Geometry: final body of the model. Coordinates: model frame, mm. A direction names the side the tool comes from. Coordinates: 2 decimals unless noted, no trailing zeros. Write each loop counter-clockwise with the first axis right and the second up, starting at its lowest first coordinate (ties: lowest second). Pieces come first, ordered by that corner, then holes. Notation, with made-up numbers: (53.5, 40.25) - (62.5, 40.25) arc R14 ccw to (62.5, 56.25) - close; hole circle Ø9 at (1.5, 83.5). An arc over 180 degrees is marked (long way). Put each result on its own line as item: value.
```python
from build123d import *

# Parameters (mm, degrees)
SKETCH1_W              = 250
SKETCH1_H              = 358.226
BASE_FLANGE1_DEPTH     = 0.91
SKETCHED_START         = -125
SKETCHED_BEND1_DEPTH   = 250
SKETCHED_BEND1_2_DEPTH = 250
SKETCH10_R             = 2.35
CUT_EXTRUDE1_DEPTH     = 0.91
FILLET1_R              = 1.5
SKETCH11_R             = 2.35
CUT_EXTRUDE2_DEPTH     = 10
SKETCH12_R             = 1.7
SKETCH12_W             = 30.3
SKETCH12_H             = 22.3
CUT_EXTRUDE3_DEPTH     = 10
FILLET2_R              = 5


# Read off the part's stored shape, not the designer's step: Sketched Bend1
# Sheet-metal steps are written as plain solids
with BuildPart() as part:
    # Sketch1 → Base-Flange1 (new body)
    with BuildSketch(Plane(origin=(0, 0, 0), x_dir=(1, 0, 0), z_dir=(0, 1, 0))):
        Rectangle(SKETCH1_W, SKETCH1_H)
    extrude(amount=-BASE_FLANGE1_DEPTH)

    # Sketched Bend1 outline → Sketched Bend1 (cut)
    with BuildSketch(Plane.YZ.offset(SKETCHED_START)):
        with BuildLine():
            ThreePointArc((-0.91, 68.830699214), (-0.668268616, 69.797195464), (0, 70.536090665))
            Line((0, 70.536090665), (0, 179.113))
            Line((0, 179.113), (-0.91, 179.113))
            Line((-0.91, 179.113), (-0.91, 68.830699214))
        make_face()
    extrude(amount=SKETCHED_BEND1_DEPTH, mode=Mode.SUBTRACT)

    # Sketched Bend1 2 outline → Sketched Bend1 2 (add)
    with BuildSketch(Plane.YZ.offset(SKETCHED_START)):
        with BuildLine():
            Line((109.086699214, 69.973699214), (109.086699214, 70.883699214))
            Line((109.086699214, 70.883699214), (1.143, 70.883699214))
            ThreePointArc((1.143, 70.883699214), (0.545655731, 70.794875587), (0, 70.536090665))
            Line((0, 70.536090665), (0, 68.830699214))
            ThreePointArc((0, 68.830699214), (0.334776949, 69.638922265), (1.143, 69.973699214))
            Line((1.143, 69.973699214), (109.086699214, 69.973699214))
        make_face()
    extrude(amount=SKETCHED_BEND1_2_DEPTH)

    # Sketch10 → Cut-Extrude1 (cut)
    with BuildSketch(Plane(origin=(0, 0, 0), x_dir=(1, 0, 0), z_dir=(0, 1, 0))):
        with Locations(Location((-105, 159.113, 0), (0, 0, 270))):
            Circle(SKETCH10_R)
        with Locations(Location((105, 159.113, 0), (0, 0, 270))):
            Circle(SKETCH10_R)
        with Locations(Location((105, -50.883699214, 0), (0, 0, 270))):
            Circle(SKETCH10_R)
        with Locations(Location((-105, -50.883699214, 0), (0, 0, 270))):
            Circle(SKETCH10_R)
    extrude(amount=-CUT_EXTRUDE1_DEPTH, mode=Mode.SUBTRACT)

    # Fillet1
    fillet1_edges = [part.edges().sort_by_distance(p)[0] for p in [
        (-125, -0.455, -179.113),
        (125, -0.455, -179.113),
        (125, 109.086699214, 70.428699214),
        (-125, 109.086699214, 70.428699214),
    ]]
    fillet(fillet1_edges, radius=FILLET1_R)

    # Sketch11 → Cut-Extrude2 (cut)
    with BuildSketch(Plane(origin=(0, 0, 0), x_dir=(1, 0, 0), z_dir=(0, 1, 0))):
        with Locations(Location((25, 124.113, 0), (0, 0, 270))):
            Circle(SKETCH11_R)
        with Locations(Location((-25, 124.113, 0), (0, 0, 270))):
            Circle(SKETCH11_R)
        with Locations(Location((-25, -25.887, 0), (0, 0, 270))):
            Circle(SKETCH11_R)
        with Locations(Location((25, -25.887, 0), (0, 0, 270))):
            Circle(SKETCH11_R)
    extrude(amount=-CUT_EXTRUDE2_DEPTH, mode=Mode.SUBTRACT)

    # Sketch12 → Cut-Extrude3 (cut)
    with BuildSketch(Plane.XY.offset(70.883699214)):
        with Locations((-20, 80)):
            Circle(SKETCH12_R)
        with Locations((20, 80)):
            Circle(SKETCH12_R)
        with Locations((0, 80)):
            Rectangle(SKETCH12_W, SKETCH12_H)
    extrude(amount=-CUT_EXTRUDE3_DEPTH, mode=Mode.SUBTRACT)

    # Fillet2
    fillet2_edges = [part.edges().sort_by_distance(p)[0] for p in [
        (15.15, 91.15, 70.428699214),
        (15.15, 68.85, 70.428699214),
        (-15.15, 68.85, 70.428699214),
        (-15.15, 91.15, 70.428699214),
    ]]
    fillet(fillet2_edges, radius=FILLET2_R)


solid = part.part
```
1. Set-up query: faces 1 (the flat face through (-2, 54, 69.974)), 2 (the flat face through (-2, -0.91, -57)). Return all of +Z, -Z, +X, -X, +Y, -Y with unobstructed straight access to the full face (end or side cutting, diameter ignored); none if empty.
Answer below:
face 1: -Z, +X, -X, +Y
face 2: +Z, -Z, +X, -X, -Y
2. Section query B-B (y = 65.5). Return loops of the section in (x, z).
Answer below:
outline: (-125, 69.97) - (125, 69.97) - (125, 70.88) - (-125, 70.88) - close
3. Pin query (flat end, axial travel): pin 1 Ø6 at (x, z) = (-25, -124.113) entering from +Y; pin 2 Ø5 at (x, y) = (-94.5, 95) entering from -Z; pin 3 Ø0.5 at (x, z) = (-3.5, 70.5) entering from -Y. Return the tip coordinate at first contact, or that it passes through.
Answer below:
pin 1: stops at y = 0
pin 2: stops at z = 69.97
pin 3: stops at y = -0.34
4. Ray query, probe 1 along Y at (x, z) = (-17.5, 53.5); probe 2 along Z at (x, y) = (111, 7.5). Return the intervals inside material, ascending. Write a range as from..to.
Answer below:
probe 1: y = -0.91..0
probe 2: z = 69.97..70.88
5. Section query A-A (x = -64.5). Return loops of the section in (y, z).
Answer below:
outline: (-0.91, -179.11) - (0, -179.11) - (0, 68.83) arc R1.14 cw to (1.14, 69.97) - (109.09, 69.97) - (109.09, 70.88) - (1.14, 70.88) arc R2.05 ccw to (-0.91, 68.83) - close
6. Section query C-C (z = -76). Return loops of the section in (x, y).
Answer below:
outline: (-125, -0.91) - (125, -0.91) - (125, 0) - (-125, 0) - close
